```python
from build123d import *
from build123d.topology import SkipClean

# Parameters (mm, degrees)
CROQUIS1_R                          = 13
CROQUIS1_R_2                        = 11.05
SALIENTE_EXTRUIR1_DEPTH             = 1
BARRER_L_MINA1_PROFILE_R            = 13.05
BARRER_L_MINA1_PROFILE_R_2          = 11.05
CROQUIS19_R                         = 13
CROQUIS19_R_2                       = 11.05
SALIENTE_EXTRUIR2_DEPTH             = 14
SALIENTE_EXTRUIR2_DIRECTION_2_REACH = 73.397
CORTAR_EXTRUIR1_START               = -32.0000001
CORTAR_EXTRUIR1_OUTLINE_R           = 11.05
CORTAR_EXTRUIR1_DEPTH               = 32.0000001


with BuildPart() as part:
    # Croquis1 → Saliente-Extruir1 (new body)
    with BuildSketch(Plane(origin=(0, 0, 0), x_dir=(1, 0, 0), z_dir=(0, 1, 0))):
        with Locations(Location((0, 0, 0), (0, 0, 270))):
            Circle(CROQUIS1_R)
        with Locations(Location((0, 0, 0), (0, 0, 270))):
            Circle(CROQUIS1_R_2, mode=Mode.SUBTRACT)
    extrude(amount=SALIENTE_EXTRUIR1_DEPTH)

    # Barrer-Lámina1: sweep along a path in Croquis2
    with BuildLine(Plane.XY) as barrer_l_mina1_path:
        Line((0, 1), (0, 21))
        ThreePointArc((0, 21), (-2.727754239, 29.625078781), (-9.918931196, 35.113211534))
        Line((-9.918931196, 35.113211534), (-29.677427344, 42.226707859))
    # Barrer-Lámina1 profile (on start of the path) → Barrer-Lámina1 (sweep)
    with BuildSketch(Plane.ZX.offset(1)):
        Circle(BARRER_L_MINA1_PROFILE_R)
        Circle(BARRER_L_MINA1_PROFILE_R_2, mode=Mode.SUBTRACT)
    sweep(path=barrer_l_mina1_path.line)

    # Croquis19 → Saliente-Extruir2 (add)
    with BuildSketch(Plane(origin=(0, 0, -18), x_dir=(-1, 0, 0), z_dir=(0, 0, -1))):
        with Locations((0, 13)):
            Circle(CROQUIS19_R)
        with Locations((0, 13)):
            Circle(CROQUIS19_R_2, mode=Mode.SUBTRACT)
    extrude(amount=SALIENTE_EXTRUIR2_DEPTH)

    # Croquis19 → Saliente-Extruir2 direction 2 (add, up to next)
    with BuildSketch(Plane(origin=(0, 0, -18), x_dir=(-1, 0, 0), z_dir=(0, 0, -1)), mode=Mode.PRIVATE) as saliente_extruir2_direction_2_sk1:
        with Locations((0, 13)):
            Circle(CROQUIS19_R)
        with Locations((0, 13)):
            Circle(CROQUIS19_R_2, mode=Mode.SUBTRACT)
    saliente_extruir2_direction_2_tool1 = extrude(saliente_extruir2_direction_2_sk1.sketch, amount=-SALIENTE_EXTRUIR2_DIRECTION_2_REACH, mode=Mode.PRIVATE) - part.part
    add(saliente_extruir2_direction_2_tool1.solids().sort_by_distance((12.632304, 13, -18))[0])

    # Cortar-Extruir1: read off the stored shape, not the designer's step
    # Cortar-Extruir1 outline → Cortar-Extruir1 (cut)
    with SkipClean():  # the faces are left unmerged after this step: merging them gives an invalid solid
        with BuildSketch(Plane(origin=(0, 0, -32), x_dir=(-1, 0, 0), z_dir=(0, 0, -1)).offset(CORTAR_EXTRUIR1_START)):
            with Locations((0, 13)):
                Circle(CORTAR_EXTRUIR1_OUTLINE_R)
        extrude(amount=CORTAR_EXTRUIR1_DEPTH, mode=Mode.SUBTRACT)


solid = part.part
```
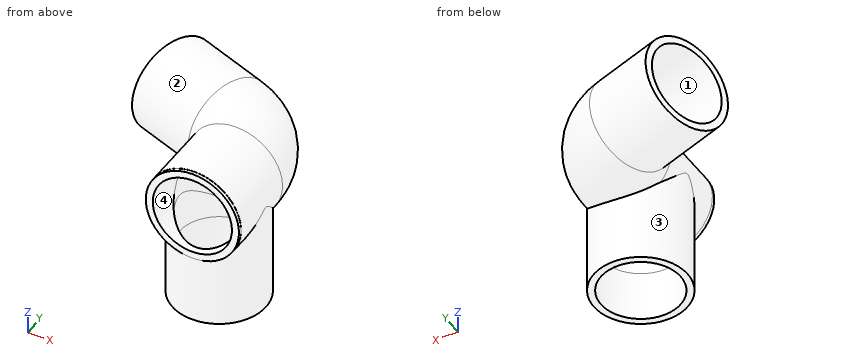
The listing builds one solid part. Answer for the finished solid, in the listing's coordinates (mm). Face numbers are marked on the shaded views. Coordinates: 2 decimals unless noted, no trailing zeros. Write each loop counter-clockwise with the first axis right and the second up, starting at its lowest first coordinate (ties: lowest second). Pieces come first, ordered by that corner, then holes. Notation, with made-up numbers: (79, 67) - (131, 67) arc R7 cw to (131, 77) - close; hole circle Ø3 at (-34, 53). An arc over 180 degrees is marked (long way). Return JSON: item names as keys, results as strings. Group by question number.
Q1. Find the intervals of material crossed by line 1 along X through (y, z) = (13, -7); line 2 along Y through (x, z) = (0, -22); line 3 along Z through (x, y) = (-1.5, 27), in increasing order. Write a range as [from, to].
Q2. The part is cut by section B-B on z = -26.5. Write down the section's boundary in (x, y).
Q3. For a pull along Z with two mould halves and no side action, classify the marked faces 1, 2, 3 and 4 as +Z half, -Z half, draft (parallel to the pull), parting line (faces both ways), or undercut.
Q4. The part is cut by section C-C on y = 7. Write down the section's boundary in (x, z), and give its area (3 significant figures).
Q5. The part is cut by section A-A on y = 13. Write down the section's boundary in (x, z).
Q6. Flat-ended cylindrical pins translate along their axes: pin 1 Ø4 at (x, z) = (-19, -11) entering from +Y; pin 2 Ø2 at (y, z) = (7.5, -8) entering from +X; pin 3 Ø6 at (y, z) = (12.5, -26.5) entering from +X. Find the tip coordinate at first contact, or state that the pin passes through.
Evaluation:
{
 "1": {"line 1": "x = [-13, -11.05], [11.05, 13]", "line 2": "y = [0, 1.95], [24.05, 26]", "line 3": "z = [-13.05, -11.05], [11.05, 13.05]"},
 "2": {"outline": "circle Ø26 at (0, 13); hole circle Ø22.1 at (0, 13)"},
 "3": {"face 1": "undercut", "face 2": "parting line", "face 3": "draft", "face 4": "undercut"},
 "4": {"outline": "(-11.53, -32) - (-9.28, -32) - (-9.28, -6) arc R11.05 cw (long way) to (9.28, -6) - (9.28, -32) - (11.53, -32) - (11.53, -6.11) arc R13.05 ccw (long way) to (-11.53, -6.11) - close", "area": "218 mm2"},
 "5": {"outline": "(-13, -32) - (-11.05, -32) - (-11.05, 0) arc R11.05 cw to (11.05, 0) - (11.05, -32) - (13, -32) - (13, -1.14) arc R13.05 ccw (long way) to (-13, -1.14) - close"},
 "6": {"pin 1": "stops at y = 48.55", "pin 2": "stops at x = 12.2", "pin 3": "stops at x = 13"}
}
